Part model, mm, in its own coordinate system. Face numbers are marked on the shaded views. A direction names the side the tool comes from. Round coordinates to 2 decimals unless told otherwise and drop trailing zeros. Loops run counter-clockwise (first coordinate to the right, second up) from the corner with the lowest first, then second, coordinate; pieces in that order, holes last. Notation, with made-up numbers: (57, 62.25) -> (99, 62.25) arc R20 ccw to (99, 78.25) -> close; hole circle Ø3 at (-7, 75). An arc over 180 degrees is marked (long way). Use a Markdown table: item, result. Add a question column.
Item 1: Cut at A-A, the plane z = -6. List the corners of the cut face in (x, y).
Item 2: Cut at B-B, the plane x = 30.4. List the corners of the cut face in (y, z).
Item 3: Cut at D-D, the plane z = -15. List the corners of the cut face in (x, y), plus the area to 3 significant figures.
Item 4: Cut at C-C, the plane y = -46. List the corners of the cut face in (x, z), plus the area to 3 significant figures.
Item 5: Flat gauge pins, fed straight in: pin 1 (1.3 mm diameter, centred on y = -10.5, z = 21, fed in from -X); pin 2 (8 mm diameter, centred on x = 23, z = -1, fed in from -Y); pin 3 (3 mm diameter, centred on x = 5.5, z = -25.5, fed in from +Y). Where does each tip first touch, or does it go through?
Item 6: Which spindle directions (+Z, -Z, +X, -X, +Y, -Y) get a long thin tool onto all of the face, cutting with end or side? Do the marked faces 1, 2 and 3. Say none if no direction does.
Item 7: Probe line 1 (Z direction, x = 23.5, y = -48); line 2 (X direction, y = -48, z = -17); line 3 (X direction, y = -0.8, z = -15). List the from-to ranges inside material, lowest first. Write a range as [from, to].
Item 8: Two-plate mould, pull along Z, no slides. Class the marked faces 4, 5 and 6: pulls with the +Z half, pulls with the -Z half, needs draft (parallel to the pull), parting line crosses it, or undercut.
```python
from build123d import *

# Parameters (mm, degrees)
F0_W     = 75.2
F0_H     = 43.2
F0_W_2   = 72
F0_H_2   = 40
F1_DEPTH = 52
F2_R     = 2
F3_DEPTH = 1.6
F5_DEPTH = 36
F6_D     = 9
F7_D     = 5
F8_W     = 1
F8_H     = 20
F9_DEPTH = 25


with BuildPart() as f1:
    # F0 (on Front) → F1 (new body)
    with BuildSketch(Plane.XZ):
        Rectangle(F0_W, F0_H)
        Rectangle(F0_W_2, F0_H_2, mode=Mode.SUBTRACT)
    extrude(amount=F1_DEPTH)

    # F2
    f2_edges = [f1.edges().sort_by_distance(p)[0] for p in [
        (37.6, -26, 21.6),
        (-37.6, -26, 21.6),
        (-37.6, -26, -21.6),
        (37.6, -26, -21.6),
    ]]
    fillet(f2_edges, radius=F2_R)

    # F0 (on Front) → F3 (join)
    with BuildSketch(Plane.XZ):
        Rectangle(F0_W_2, F0_H_2)
    extrude(amount=F3_DEPTH)

    # F4 (on Right) → F5 (join, symmetric)
    with BuildSketch(Plane.YZ):
        Polygon((0, -21.6), (-52, -21.6), (-41.0421315348, -42.8069394041), align=None)
    extrude(amount=F5_DEPTH, both=True)

    # F6 (through all)
    with Locations(Plane(origin=(0, 0, 0), x_dir=(1, 0, 0), z_dir=(0, 1, 0))):
        with Locations((30.4, 6)):
            Hole(F6_D / 2)

    # F7 (through all)
    with Locations(Plane(origin=(0, 0, 0), x_dir=(1, 0, 0), z_dir=(0, 1, 0))):
        with Locations((-6, 15)):
            Hole(F7_D / 2)

    # F8 (on face) → F9 (cut)
    with BuildSketch(Plane.XY.offset(21.6)):
        with Locations((-32.2436588705, -14.5910207555)):
            Rectangle(F8_W, F8_H)
        with Locations((-28.8436588705, -14.5910207555)):
            Rectangle(F8_W, F8_H)
        with Locations((-25.4436588705, -14.5910207555)):
            Rectangle(F8_W, F8_H)
        with Locations((-22.0436588705, -14.5910207555)):
            Rectangle(F8_W, F8_H)
        with Locations((-18.6436588705, -14.5910207555)):
            Rectangle(F8_W, F8_H)
        with Locations((-15.2436588705, -14.5910207555)):
            Rectangle(F8_W, F8_H)
        with Locations((-11.8436588705, -14.5910207555)):
            Rectangle(F8_W, F8_H)
        with Locations((-8.4436588705, -14.5910207555)):
            Rectangle(F8_W, F8_H)
        with Locations((-5.0436588705, -14.5910207555)):
            Rectangle(F8_W, F8_H)
        with Locations((1.7563411295, -14.5910207555)):
            Rectangle(F8_W, F8_H)
        with Locations((5.1563411295, -14.5910207555)):
            Rectangle(F8_W, F8_H)
        with Locations((-1.6436588705, -14.5910207555)):
            Rectangle(F8_W, F8_H)
        with Locations((8.5563411295, -14.5910207555)):
            Rectangle(F8_W, F8_H)
        with Locations((11.9563411295, -14.5910207555)):
            Rectangle(F8_W, F8_H)
        with Locations((15.3563411295, -14.5910207555)):
            Rectangle(F8_W, F8_H)
        with Locations((18.7563411295, -14.5910207555)):
            Rectangle(F8_W, F8_H)
        with Locations((22.1563411295, -14.5910207555)):
            Rectangle(F8_W, F8_H)
        with Locations((25.5563411295, -14.5910207555)):
            Rectangle(F8_W, F8_H)
        with Locations((28.9563411295, -14.5910207555)):
            Rectangle(F8_W, F8_H)
        with Locations((32.3563411295, -14.5910207555)):
            Rectangle(F8_W, F8_H)
    extrude(amount=-F9_DEPTH, mode=Mode.SUBTRACT)


solid = f1.part
```
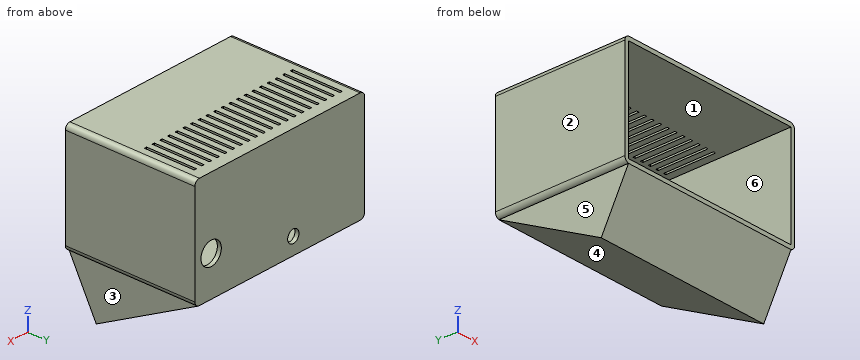
A:
| question | item | result |
|---|---|---|
| 1 | outline | (-37.6, -52) -> (-36, -52) -> (-36, -1.6) -> (25.9, -1.6) -> (25.9, 0) -> (-37.6, 0) -> close; (34.9, -1.6) -> (36, -1.6) -> (36, -52) -> (37.6, -52) -> (37.6, 0) -> (34.9, 0) -> close |
| 2 | outline | (-52, -21.6) -> (-41.04, -42.81) -> (0, -21.6) -> (0, -10.5) -> (-1.6, -10.5) -> (-1.6, -20) -> (-52, -20) -> close; (-52, 20) -> (-1.6, 20) -> (-1.6, -1.5) -> (0, -1.5) -> (0, 21.6) -> (-52, 21.6) -> close |
| 3 | outline | (-37.6, -52) -> (-36, -52) -> (-36, -1.6) -> (-8.5, -1.6) -> (-8.5, 0) -> (-37.6, 0) -> close; (-3.5, -1.6) -> (36, -1.6) -> (36, -52) -> (37.6, -52) -> (37.6, 0) -> (-3.5, 0) -> close |
| 3 | area | 274 mm^2 |
| 4 | outline | (-37.6, -19.6) arc R2 ccw to (-35.6, -21.6) -> (-36, -21.6) -> (-36, -33.21) -> (36, -33.21) -> (36, -21.6) -> (35.6, -21.6) arc R2 ccw to (37.6, -19.6) -> (37.6, 19.6) arc R2 ccw to (35.6, 21.6) -> (-35.6, 21.6) arc R2 ccw to (-37.6, 19.6) -> close; hole (-36, -20) -> (36, -20) -> (36, 20) -> (-36, 20) -> close |
| 4 | area | 1,200 mm^2 |
| 5 | pin 1 | stops at x = -37.45 |
| 5 | pin 2 | stops at y = -1.6 |
| 5 | pin 3 | stops at y = -4.64 |
| 6 | face 1 | -Y |
| 6 | face 2 | +Z, -Z, -X, +Y, -Y |
| 6 | face 3 | -Z, +X, +Y, -Y |
| 7 | line 1 | z = [-29.34, -20], [20, 21.6] |
| 7 | line 2 | x = [-37.6, -36], [36, 37.6] |
| 7 | line 3 | x = [-37.6, -8.5], [-3.5, 37.6] |
| 8 | face 4 | pulls with the -Z half |
| 8 | face 5 | needs draft |
| 8 | face 6 | undercut |
